Check sheet for the drawn part. Datum: minimum x, y, z corner. Units: mm. Give positions to 0.01 mm unless a question says otherwise; leave off trailing zeros. Loops run counter-clockwise (first coordinate to the right, second up) from the corner with the lowest first, then second, coordinate; pieces in that order, holes last. Notation, with made-up numbers: (37, 52.5) - (46, 52.5) arc R24 ccw to (46, 69.5) - close; hole circle Ø7 at (56.25, 71). An arc over 180 degrees is marked (long way). Use one line per item in the form item = value.
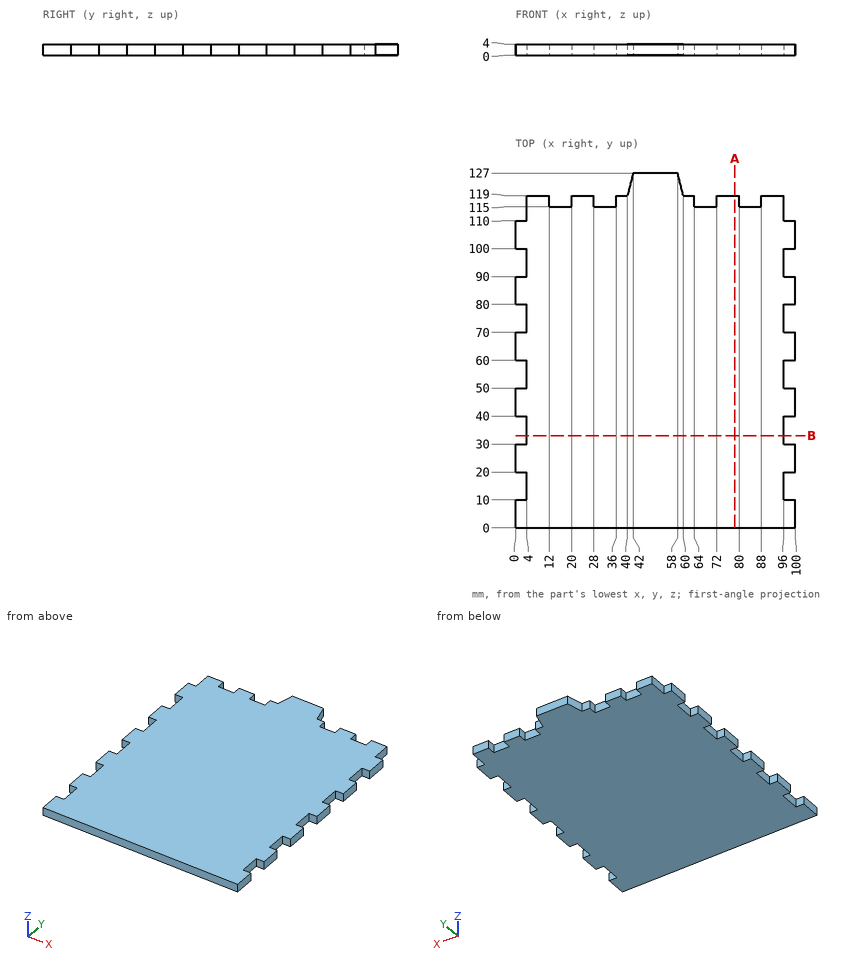
Item 1: Gauge pin test, flat ends, axial feed: P1, Ø1.2, axis at x = 2, z = 2.5, coming from the +Y side; P2, Ø1, axis at x = 32.5, z = 2, coming from the +Y side; P3, Ø1.2, axis at x = 92, z = 3, coming from the +Y side. Record the tip position at first contact, or that the pin passes through.
Answer block:
P1 = 110
P2 = 115
P3 = 119
Item 2: Section check A-A on x = 78.5. Record the boundary of the cut face in (y, z), then the cut area to 3 significant figures.
Answer block:
outline = (0, 0) - (119, 0) - (119, 4) - (0, 4) - close
area = 476 mm2
Item 3: Thickness scan on L1, parallel to Y at x = 86, z = 3.6; L2, parallel to Y at x = 9.5, z = 0.35; L3, parallel to X at y = 78, z = 0.25. Record the ranges inside material, lowest first.
Answer block:
L1 = 0 to 115
L2 = 0 to 119
L3 = 4 to 96
Item 4: Section check B-B on y = 33. Record the boundary of the cut face in (x, z), then the cut area to 3 significant figures.
Answer block:
outline = (4, 0) - (96, 0) - (96, 4) - (4, 4) - close
area = 368 mm2
